```python
from build123d import *

# Parameters (mm, degrees)
BOSS_EXTRUDE1_DEPTH = 5
SKETCH2_R           = 5
CUT_EXTRUDE1_DEPTH  = 10
SKETCH3_W           = 30
SKETCH3_H           = 30
BOSS_EXTRUDE2_DEPTH = 5
BOSS_EXTRUDE3_DEPTH = 5
SKETCH6_R           = 5
CUT_EXTRUDE2_DEPTH  = 5
SKETCH7_W           = 46.54134698
SKETCH7_H           = 34.044615897
CUT_EXTRUDE3_DEPTH  = 5


with BuildPart() as part:
    # Sketch1 → Boss-Extrude1 (new body)
    with BuildSketch(Plane.XY):
        with BuildLine():
            Line((5, 0), (70, 0))
            Line((70, 0), (70, -30))
            Line((70, -30), (70, -95))
            Line((70, -95), (40, -95))
            Line((40, -95), (40, -30))
            Line((40, -30), (5, -30))
            ThreePointArc((5, -30), (1.464466094, -28.535533906), (0, -25))
            Line((0, -25), (0, -5))
            ThreePointArc((0, -5), (1.464466094, -1.464466094), (5, 0))
        make_face()
    boss_extrude1 = extrude(amount=BOSS_EXTRUDE1_DEPTH)

    # Sketch2 → Cut-Extrude1 (cut)
    with BuildSketch(Plane.XY.offset(5)):
        with Locations((15, -15)):
            Circle(SKETCH2_R)
    extrude(amount=-CUT_EXTRUDE1_DEPTH, mode=Mode.SUBTRACT)

    # Sketch3 → Boss-Extrude2 (add)
    with BuildSketch(Plane.XZ.offset(95)):
        with Locations((55, 15)):
            Rectangle(SKETCH3_W, SKETCH3_H)
    extrude(amount=BOSS_EXTRUDE2_DEPTH)

    # Sketch4 → Boss-Extrude3 (add)
    with BuildSketch(Plane.ZY.offset(-40)):
        Polygon((5, -70), (30, -95), (5, -95), align=None)
    boss_extrude3 = extrude(amount=-BOSS_EXTRUDE3_DEPTH)

    # Mirror1: Boss-Extrude3 across plane
    add(boss_extrude3.mirror(Plane.ZY.offset(-55)))

    # Mirror2: Boss-Extrude1 across plane
    add(boss_extrude1.mirror(Plane.ZY.offset(-55)))

    # Sketch6 → Cut-Extrude2 (cut)
    with BuildSketch(Plane.XY.offset(5)):
        with Locations((95, -15)):
            Circle(SKETCH6_R)
    extrude(amount=-CUT_EXTRUDE2_DEPTH, mode=Mode.SUBTRACT)

    # Sketch7 → Cut-Extrude3 (cut)
    with BuildSketch(Plane.XY.offset(5)):
        with Locations((16.72932651, -12.977692052)):
            Rectangle(SKETCH7_W, SKETCH7_H)
    extrude(amount=-CUT_EXTRUDE3_DEPTH, mode=Mode.SUBTRACT)


solid = part.part
```
For this review, take the finished solid that the model builds, in its own axes (mm). A direction names the side the tool comes from. Coordinates: 2 decimals unless noted, no trailing zeros. Loops run counter-clockwise (first coordinate to the right, second up) from the corner with the lowest first, then second, coordinate; pieces in that order, holes last.
1. For faces 4 (the flat face through (87, -30, 2)), 5 (the flat face through (65, -88, 12)), 6 (the flat face through (68, -82, 17)), list the 3-axis set-ups (+Z, -Z, +X, -X, +Y, -Y) from which the entire face can be reached by the end or side of a thin tool; tool diameter is ignored.
2. Insertion check: P1, Ø1, axis at x = 71, z = 5, coming from the +Y side; P2, Ø1, axis at x = 48, y = -52.5, coming from the +Z side; P3, Ø8, axis at x = 76, z = 22, coming from the +Y side; P4, Ø12.5, axis at y = -79, z = 22, coming from the +X side. Each pin has a flat end and moves straight along its axis. Give the tip position at first contact, or say it passes through.
3. Add section D-D, the plane y = -88. Give the boundary of the cut face in (x, z), then the cut area to 3 significant figures.
4. Add section A-A, the plane x = 95. Give the boundary of the cut face in (y, z), then the cut area to 3 significant figures.
5. Mouldability with a two-part tool opening along X and no side actions: class faces 1 (the flat face through (45, -88, 12)), 2 (the flat face through (67, -38, 0)), 3 (the cylindrical face through (109, -2, 2)) as +X half, -X half, draft (parallel to the pull), parting line (faces both ways), or undercut.
6. Add section B-B, the plane y = -15. Give the boundary of the cut face in (x, z), then the cut area to 3 significant figures.
7. For line 1 (Y direction, x = 95, z = 1.4); line 2 (Y direction, x = 60.5, z = 10); line 3 (X direction, y = -16.5, z = 4), list the stretches that pass through material, from the lowest coordinate up.
8. Add section C-C, the plane z = 18.5. Give the boundary of the cut face in (x, y), then the cut area to 3 significant figures.
Result:
1. face 4: +Z, -Z, +X, -Y
1. face 5: +Z, +Y
1. face 6: +Z, +X, -X, +Y
2. P1: stops at y = 0
2. P2: stops at z = 5
2. P3: passes through
2. P4: stops at x = 70
3. outline: (40, 0) - (70, 0) - (70, 23) - (65, 23) - (65, 5) - (45, 5) - (45, 23) - (40, 23) - close
3. area: 330 mm2
4. outline: (-30, 0) - (-20, 0) - (-20, 5) - (-30, 5) - close; (-10, 0) - (0, 0) - (0, 5) - (-10, 5) - close
4. area: 100 mm2
5. face 1: undercut
5. face 2: draft
5. face 3: +X half
6. outline: (40, 0) - (90, 0) - (90, 5) - (40, 5) - close; (100, 0) - (110, 0) - (110, 5) - (100, 5) - close
6. area: 300 mm2
7. line 1: y = -30 to -20, -10 to 0
7. line 2: y = -100 to -95
7. line 3: x = 40 to 90.23, 99.77 to 110
8. outline: (40, -100) - (70, -100) - (70, -83.5) - (65, -83.5) - (65, -95) - (45, -95) - (45, -83.5) - (40, -83.5) - close
8. area: 265 mm2
